For this review, take the finished solid that the model builds, in its own axes (mm). Face numbers are marked on the shaded views. A direction names the side the tool comes from. Give positions to 0.01 mm unless a question says otherwise; leave off trailing zeros. Write each loop counter-clockwise with the first axis right and the second up, starting at its lowest first coordinate (ties: lowest second). Pieces come first, ordered by that corner, then holes.
Autodesk Fusion 360 part; units mm, degrees
sketch "Sketch1" plane through (0, 0, 0) normal (0, 0, 1) x (1, 0, 0)
sketch "Sketch2" plane through (0, 0, 0) normal (0, 1, 0) x (1, 0, 0)
  line L0 (0, 0) -> (-16, 0)
  line L1 (-16, 0) -> (-16, -5)
  line L2 (-16, -5) -> (0, -5)
  line L3 (0, -5) -> (0, 0)
  line L4 (0, 0) -> (-5, 0)
  line L5 (-5, 0) -> (-5, -25)
  line L6 (-5, -25) -> (0, -25)
  line L7 (0, -25) -> (0, 0)
  dimension "d1" = 16
  dimension "d2" = 5
  dimension "d3" = 5
  dimension "d4" = 25
extrude "Extrude1" add sketch "Sketch2" along normal blind 50
sketch "Sketch3" plane through (-5, 0, 0) normal (-1, 0, 0) x (0, -1, 0)
  line L0 (0, 5) -> (0, 25)
  line L1 (0, 25) -> (-50, 25)
  line L2 (-50, 25) -> (-50, 5)
  line L3 (-50, 5) -> (0, 5)
  line L4 (-50, 5) -> (-45, 5)
  line L5 (-45, 5) -> (-5, 5)
  line L6 (-5, 5) -> (-5, 20)
  line L7 (-5, 20) -> (-45, 20)
  line L8 (-45, 20) -> (-45, 5)
  dimension "d7" = 5
  dimension "d8" = 40
  dimension "d9" = 15
extrude "Extrude2" cut sketch "Sketch3" against normal blind 1000 contours L3 L5 L6 L7 L8
sketch "Sketch4" plane through (0, 0, 25) normal (0, 0, 1) x (-1, 0, 0)
  line L0 (5, 0) -> (0, 0)
  line L1 (0, 0) -> (0, -50)
  line L2 (0, -50) -> (5, -50)
  line L3 (5, -50) -> (5, 0)
  line L4 (0, -50) -> (0, -48.675)
  line L5 (0, -48.675) -> (1.325, -48.675)
  line L6 (1.325, -48.675) -> (3.625, -48.675)
  line L7 (3.625, -48.675) -> (3.625, -46.375)
  line L8 (3.625, -46.375) -> (1.325, -46.375)
  line L9 (1.325, -46.375) -> (1.325, -48.675)
  line L10 (0, 0) -> (0, -1.325)
  line L11 (0, -1.325) -> (1.325, -1.325)
  line L12 (1.325, -1.325) -> (3.625, -1.325)
  line L13 (3.625, -1.325) -> (3.625, -3.625)
  line L14 (3.625, -3.625) -> (1.325, -3.625)
  line L15 (1.325, -3.625) -> (1.325, -1.325)
  dimension "d12" = 1.325
  dimension "d13" = 1.325
  dimension "d14" = 2.3
  dimension "d15" = 2.3
  dimension "d16" = 1.325
  dimension "d17" = 1.325
  dimension "d18" = 2.3
  dimension "d19" = 2.3
extrude "Extrude3" cut sketch "Sketch4" against normal blind 5
sketch "Sketch5" plane through (0, 0, 5) normal (0, 0, 1) x (-1, 0, 0)
  line L0 (16, 0) -> (5, 0)
  line L1 (5, 0) -> (5, -5)
  line L2 (5, -5) -> (0, -5)
  line L3 (0, -5) -> (0, -45)
  line L4 (0, -45) -> (5, -45)
  line L5 (5, -45) -> (5, -50)
  line L6 (5, -50) -> (16, -50)
  line L7 (16, -50) -> (16, 0)
  line L8 (8, -50) -> (8, -25)
  line L9 (8, -25) -> (8, -32.25)
  line L10 (8, -32.25) -> (8, -17.75)
  line L11 (0, -36) -> (7.25, -36)
  line L12 (7.25, -36) -> (7.25, -31.1746)
  line L13 (8, -32.25) -> (7.25, -32.25)
  line L14 (7.25, -32.25) -> (8, -32.25)
  circle A0 centre (8, -32.25) radius 0.75
  line L15 (8, -32.25) -> (8, -17.75)
  circle A1 centre (8, -17.75) radius 0.75
  dimension "d22" = 25
  dimension "d23" = 7.25
  dimension "d24" = 14.5
  dimension "d25" = 7.25
  dimension "d26" = 0.75
  dimension "d27" = 1.5
  dimension "d28" = 14.5
  dimension "d29" = 1.5
extrude "Extrude4" cut sketch "Sketch5" against normal blind 1000 contours A1 | L8 L13 L14 A0 | L8 L9 L10 A0 L15 | L8 L9 L10 L13 L14 A0 L15
extrude "Extrude5" cut 2 faces at (-2.0917, 47.9083, 25) (-2.0917, 2.8583, 25) along direction (0, 0, -1) blind 5
sketch "Sketch6" plane through (0, 0, 20) normal (0, 0, 1) x (-1, 0, 0)
  line L0 (5, -45) -> (0, -45)
  line L1 (0, -45) -> (0, -50)
  line L2 (0, -50) -> (5, -50)
  line L3 (5, -50) -> (5, -45)
  line L4 (5, 0) -> (3.65, 0)
  line L5 (3.65, 0) -> (3.65, -1.35)
  line L6 (3.65, -1.35) -> (5, -1.35)
  line L7 (5, -1.35) -> (5, 0)
  line L8 (3.65, -1.35) -> (1.35, -1.35)
  line L9 (1.35, -1.35) -> (1.35, -3.65)
  line L10 (1.35, -3.65) -> (3.65, -3.65)
  line L11 (3.65, -3.65) -> (3.65, -1.35)
  line L12 (5, -45) -> (3.65, -45)
  line L13 (3.65, -45) -> (3.65, -46.35)
  line L14 (3.65, -46.35) -> (5, -46.35)
  line L15 (5, -46.35) -> (5, -45)
  line L16 (3.65, -46.35) -> (1.35, -46.35)
  line L17 (1.35, -46.35) -> (1.35, -48.65)
  line L18 (1.35, -48.65) -> (3.65, -48.65)
  line L19 (3.65, -48.65) -> (3.65, -46.35)
  dimension "d34" = 1.35
  dimension "d35" = 1.35
  dimension "d36" = 2.3
  dimension "d37" = 2.3
  dimension "d38" = 1.35
  dimension "d39" = 1.35
  dimension "d40" = 2.3
  dimension "d41" = 2.3
extrude "Extrude6" add sketch "Sketch6" along normal blind 5 contours L16 L17 L18 L19 | L8 L9 L10 L11
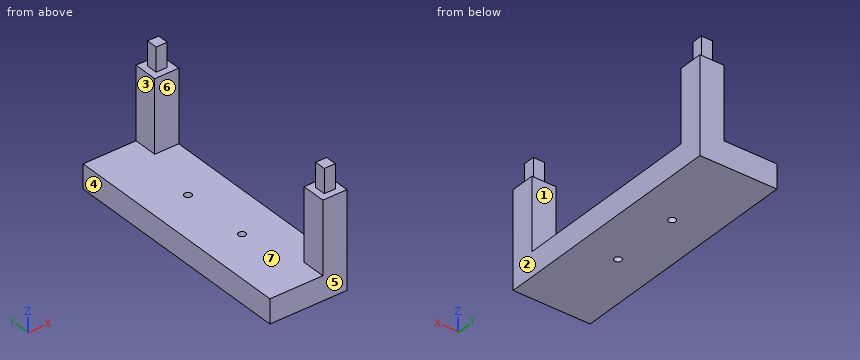
(1) We need section A-A (x = -8). Write out the cut boundary in (y, z).
(2) We need section D-D (y = 26). Write out the cut boundary in (x, z), and give its area (3 significant figures).
(3) We need section B-B (y = 17.75). Write out the cut boundary in (x, z).
(4) We need section C-C (z = 15.5). Write out the cut boundary in (x, y).
(5) Clearance check with flat-ended pins moving along their axes: pin 1 Ø2.5 at (y, z) = (48, 23) entering from -X; pin 2 Ø2.5 at (x, z) = (-2, 21.5) entering from -Y; pin 3 Ø5 at (x, y) = (-6, 19.5) entering from +Z; pin 4 Ø4 at (x, z) = (-5.5, 7.5) entering from +Y. State where each tip first meets the part, or that it passes through.
(6) For L1, parallel to Y at x = -8, z = 3.1; L2, parallel to Y at x = -3, z = 21.5; L3, parallel to X at y = 17.75, z = 2.6, list the stretches that pass through material, from the lowest coordinate up.
(7) The part is to be moulded in two halves that separate along Y. For the marked faces 4, 5, 6 and 7, say which applies: +Y half, -Y half, draft (parallel to the pull), parting line (faces both ways), or undercut.
(8) Tool access review of the marked faces 1, 2 and 3: name each direction out of +Z, -Z, +X, -X, +Y, -Y from which nothing blocks a thin tool from reaching the whole face with its end or side.
The answers:
1. outline: (0, 0) - (17, 0) - (17, 5) - (0, 5) - close; (18.5, 0) - (31.5, 0) - (31.5, 5) - (18.5, 5) - close; (33, 0) - (50, 0) - (50, 5) - (33, 5) - close
2. outline: (-16, 0) - (0, 0) - (0, 5) - (-16, 5) - close
2. area: 80.0 mm2
3. outline: (-16, 0) - (-8.75, 0) - (-8.75, 5) - (-16, 5) - close; (-7.25, 0) - (0, 0) - (0, 5) - (-7.25, 5) - close
4. outline: (-5, 0) - (0, 0) - (0, 5) - (-5, 5) - close; (-5, 45) - (0, 45) - (0, 50) - (-5, 50) - close
5. pin 1: stops at x = -3.65
5. pin 2: stops at y = 1.35
5. pin 3: stops at z = 5
5. pin 4: stops at y = 50
6. L1: y = 0 to 17, 18.5 to 31.5, 33 to 50
6. L2: y = 1.35 to 3.65, 46.35 to 48.65
6. L3: x = -16 to -8.75, -7.25 to 0
7. face 4: draft
7. face 5: -Y half
7. face 6: undercut
7. face 7: undercut
8. face 1: +Z, +X, -X
8. face 2: +Z, -Z, +X, +Y, -Y
8. face 3: +Z, -X, +Y, -Y
